Could you check a few things on this drawing? It's one solid part, dimensions in mm from its lowest x, y, z. A direction names the side the tool comes from. Coordinates: 2 decimals unless noted, no trailing zeros. Write each loop counter-clockwise with the first axis right and the second up, starting at its lowest first coordinate (ties: lowest second). Pieces come first, ordered by that corner, then holes.
Item 1: I want a section at D-D (y = 29.5). Please give me the cut outline in (x, z) (1 decimal), and give its area (3 significant figures).
Item 2: If we mould it in two halves opening along Y, with no side actions, what happens to the marked faces 1, 2, 3 and 4? For each: pulls with the +Y half, pulls with the -Y half, needs draft (parallel to the pull), parting line crosses it, or undercut.
Item 3: Please list where these lines run through material, in increasing order: line 1 (Y direction, x = 42.75, z = 4.35); line 2 (Y direction, x = 57.75, z = 3.25); line 3 (X direction, y = 44.5, z = 9.25).
Item 4: I want a section at A-A (z = 4.25). Please give me the cut outline in (x, y), and give its area (3 significant figures).
Item 5: For the marked faces 5 and 6, which set-ups out of +Z, -Z, +X, -X, +Y, -Y let a thin tool reach every point of the face, with its end or its side?
Item 6: I'm going to push flat-ended pins straight in: P1, Ø3, axis at x = 42.5, y = 44, coming from the +Z side; P2, Ø1, axis at x = 35.5, z = 5.5, coming from the -Y side; P3, Ø6.5, axis at y = 58.5, z = 10, coming from the -X side; P4, Ø3.5, axis at x = 27.75, y = 37.75, coming from the +Z side. Where does each tip first touch, or does it pass through?
Item 7: I want a section at C-C (x = 57.75). Please give me the cut outline in (y, z), and give its area (3 significant figures).
Item 8: I want a section at B-B (z = 9.5). Count the separate pieces of the cut face and the enclosed holes in it, and give its area (3 significant figures).
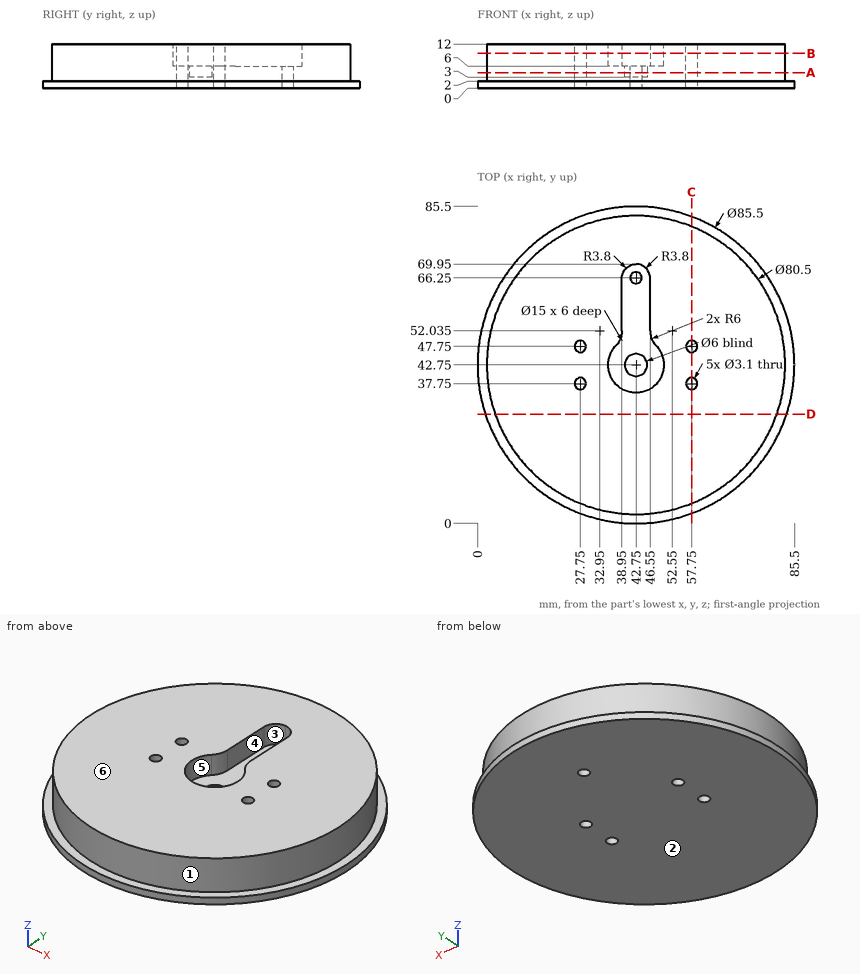
Answer:
1. outline: (2.1, 0) - (83.4, 0) - (83.4, 2) - (80.8, 2) - (80.8, 12) - (4.7, 12) - (4.7, 2) - (2.1, 2) - close
1. area: 923 mm2
2. face 1: parting line crosses it
2. face 2: needs draft
2. face 3: undercut
2. face 4: undercut
3. line 1: y = 2.5 to 39.75, 45.75 to 64.7, 67.8 to 83
3. line 2: y = 5.4 to 36.2, 39.3 to 46.2, 49.3 to 80.1
3. line 3: x = 2.54 to 35.46, 50.04 to 82.96
4. outline: circle Ø80.5 at (42.75, 42.75); hole circle Ø3.1 at (27.75, 37.75); hole circle Ø3.1 at (27.75, 47.75); hole circle Ø6 at (42.75, 42.75); hole circle Ø3.1 at (42.75, 66.25); hole circle Ø3.1 at (57.75, 37.75); hole circle Ø3.1 at (57.75, 47.75)
4. area: 5,020 mm2
5. face 5: +Z
5. face 6: +Z, +X, -X, +Y, -Y
6. P1: stops at z = 3
6. P2: stops at y = 3.07
6. P3: stops at x = 4.49
6. P4: stops at z = 12
7. outline: (2.72, 0) - (36.2, 0) - (36.2, 12) - (5.4, 12) - (5.4, 2) - (2.72, 2) - close; (39.3, 0) - (46.2, 0) - (46.2, 12) - (39.3, 12) - close; (49.3, 0) - (82.78, 0) - (82.78, 2) - (80.1, 2) - (80.1, 12) - (49.3, 12) - close
7. area: 833 mm2
8. separate pieces: 1
8. enclosed holes: 5
8. area: 4,730 mm2
